from build123d import *

# Parameters (mm, degrees)
F0_W     = 70
F0_H     = 120
F1_DEPTH = 25
F2_R     = 8
F3_DEPTH = 70
F4_R     = 5
F5_R     = 7.5


with BuildPart() as f1:
    # F0 (on Top) → F1 (new body)
    with BuildSketch(Plane.XY):
        Rectangle(F0_W, F0_H)
    extrude(amount=F1_DEPTH)

    # F2 (on face) → F3 (cut, through all)
    with BuildSketch(Plane.YZ.offset(35)):
        with Locations((-60, 25)):
            Circle(F2_R)
    extrude(amount=-F3_DEPTH, mode=Mode.SUBTRACT)

    # F4
    f4_edges = [f1.edges().sort_by_distance(p)[0] for p in [
        (0, -52, 25),
    ]]
    fillet(f4_edges, radius=F4_R)

    # F5
    f5_edges = [f1.edges().sort_by_distance(p)[0] for p in [
        (0, -60, 17),
    ]]
    fillet(f5_edges, radius=F5_R)


solid = f1.part
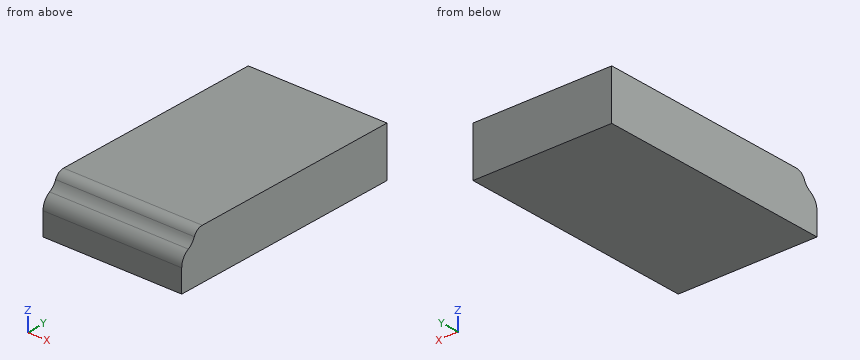
Part model, mm, in its own coordinate system. Coordinates: 2 decimals unless noted, no trailing zeros. Write each loop counter-clockwise with the first axis right and the second up, starting at its lowest first coordinate (ties: lowest second). Pieces come first, ordered by that corner, then holes. Notation, with made-up numbers: (74, -31) - (82, -31) arc R21 cw to (82, -10) - close; hole circle Ø11 at (75.5, 87.25). An arc over 180 degrees is marked (long way). Put each result on its own line as item: value.
1. Probe line 1 along Y through (x, z) = (29.5, 18); line 2 along Y through (x, z) = (25, 14); line 3 along Z through (x, y) = (0.5, -49.5). List the from-to ranges inside material, lowest first. Write a range as [from, to].
Final values:
line 1: y = [-56.13, 60]
line 2: y = [-59.55, 60]
line 3: z = [0, 24.77]
2. Band-saw the part on A-A (x = 8). Write the cut outline in (y, z).
Final values:
outline: (-60, 0) - (60, 0) - (60, 25) - (-48, 25) arc R5 ccw to (-52.62, 21.92) arc R8 cw to (-56.13, 18) arc R7.5 ccw to (-60, 11.44) - close
3. Flat gauge pin, fed straight in: pin 1 Ø3 at (x, z) = (14.5, 21.5) entering from -Y (3 decimals). Where does the tip first touch, or does it go through?
Final values:
pin 1: stops at y = -53.755
